Check sheet for the drawn part. Datum: minimum x, y, z corner. Units: mm. Give positions to 0.01 mm unless a question says otherwise; leave off trailing zeros. Loops run counter-clockwise (first coordinate to the right, second up) from the corner with the lowest first, then second, coordinate; pieces in that order, holes last. Notation, with made-up numbers: (-25, -21.75) - (27, -21.75) arc R13 ccw to (27, -6.75) - close; hole circle Ø3 at (-32.5, 28). An arc over 180 degrees is marked (long way). Answer in a Markdown table with one row per item.
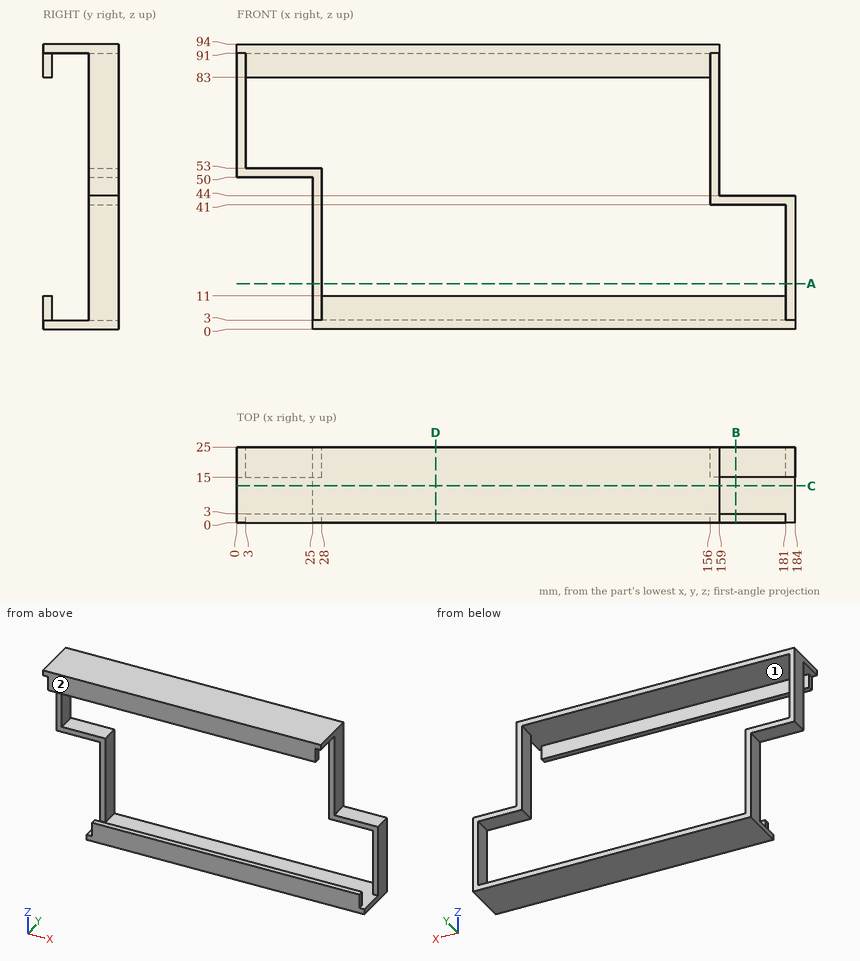
Q1. Sectioned sample at B-B (x = 164.5). Record the cut outline in (y, z), and give its area (3 significant figures).
Completed:
| item | result |
|---|---|
| outline | (0, 0) - (25, 0) - (25, 3) - (3, 3) - (3, 11) - (0, 11) - close; (15, 41) - (25, 41) - (25, 44) - (15, 44) - close |
| area | 129 mm^2 |
Q2. Sectioned sample at A-A (z = 15). Record the cut outline in (x, y).
Completed:
| item | result |
|---|---|
| outline | (25, 15) - (28, 15) - (28, 25) - (25, 25) - close; (181, 15) - (184, 15) - (184, 25) - (181, 25) - close |
Q3. Thickness scan on line 1 (Z direction, x = 45, y = 4.5); line 2 (X direction, y = 19.5, z = 75.5); line 3 (X direction, y = 22, z = 32). Record the ranges inside material, lowest first.
Completed:
| item | result |
|---|---|
| line 1 | 0 to 3, 91 to 94 |
| line 2 | 0 to 3, 156 to 159 |
| line 3 | 25 to 28, 181 to 184 |
Q4. Go/stop test with flat-tipped pins: P1, Ø6.5, axis at x = 43, z = 87.5, coming from the +Y side; P2, Ø3, axis at y = 17.5, z = 71, coming from the +X side; P3, Ø3, axis at x = 169, y = 18.5, coming from the +Z side. Record where each tip stops, or that it passes through.
Completed:
| item | result |
|---|---|
| P1 | y = 3 |
| P2 | x = 159 |
| P3 | z = 44 |
Q5. Sectioned sample at C-C (y = 12.25). Record the cut outline in (x, z), and give its area (3 significant figures).
Completed:
| item | result |
|---|---|
| outline | (0, 91) - (159, 91) - (159, 94) - (0, 94) - close; (25, 0) - (184, 0) - (184, 3) - (25, 3) - close |
| area | 954 mm^2 |
Q6. Draft check along X on the marked faces 1 and 2. Enter one of: +X half, -X half, draft (parallel to the pull), parting line (faces both ways), or undercut.
Completed:
| item | result |
|---|---|
| face 1 | undercut |
| face 2 | draft |
Q7. Sectioned sample at D-D (x = 65.5). Record the cut outline in (y, z), and give its area (3 significant figures).
Completed:
| item | result |
|---|---|
| outline | (0, 0) - (25, 0) - (25, 3) - (3, 3) - (3, 11) - (0, 11) - close; (0, 83) - (3, 83) - (3, 91) - (25, 91) - (25, 94) - (0, 94) - close |
| area | 198 mm^2 |
